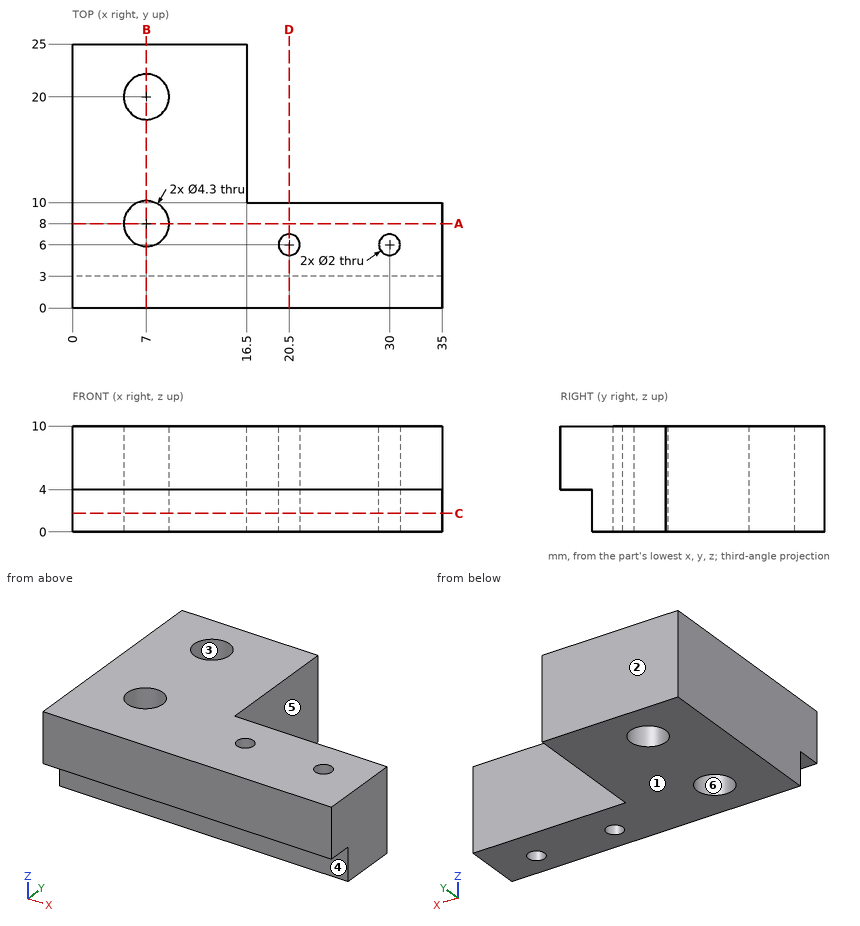
Geometry check sheet. Reference: drawing and pictorial views, mm from the part's lowest x, y, z. A direction names the side the tool comes from. Coordinates: 2 decimals unless noted, no trailing zeros. Order: outer loops, then holes, each group sorted by start corner. A loop starts at its lowest first (then second) coordinate and runs counter-clockwise, first axis right, second up.
Item 1: Section check A-A, the plane y = 8. Enter the section's corners in (x, z).
Filled in:
outline: (0, 0) - (4.85, 0) - (4.85, 10) - (0, 10) - close; (9.15, 0) - (35, 0) - (35, 10) - (9.15, 10) - close
Item 2: Material ranges on L1, parallel to Y at x = 7, z = 3; L2, parallel to Y at x = 30, z = 4.25; L3, parallel to Y at x = 8, z = 4.75, recorded low to high.
Filled in:
L1: y = 3 to 5.85, 10.15 to 17.85, 22.15 to 25
L2: y = 0 to 5, 7 to 10
L3: y = 0 to 6.1, 9.9 to 18.1, 21.9 to 25
Item 3: Section check B-B, the plane x = 7. Enter the section's corners in (y, z), then the cut area to 3 significant figures.
Filled in:
outline: (0, 4) - (3, 4) - (3, 0) - (5.85, 0) - (5.85, 10) - (0, 10) - close; (10.15, 0) - (17.85, 0) - (17.85, 10) - (10.15, 10) - close; (22.15, 0) - (25, 0) - (25, 10) - (22.15, 10) - close
area: 152 mm2
Item 4: Section check D-D, the plane x = 20.5. Enter the section's corners in (y, z).
Filled in:
outline: (0, 4) - (3, 4) - (3, 0) - (5, 0) - (5, 10) - (0, 10) - close; (7, 0) - (10, 0) - (10, 10) - (7, 10) - close
Item 5: Section check C-C, the plane z = 1.75. Enter the section's corners in (x, y), then the cut area to 3 significant figures.
Filled in:
outline: (0, 3) - (35, 3) - (35, 10) - (16.5, 10) - (16.5, 25) - (0, 25) - close; hole circle Ø4.3 at (7, 8); hole circle Ø4.3 at (7, 20); hole circle Ø2 at (20.5, 6); hole circle Ø2 at (30, 6)
area: 457 mm2
Item 6: Depth check by flat-ended pin: pin 1 (4.5 mm diameter, centred on x = 12, z = 1.5, fed in from -Y); pin 2 (4 mm diameter, centred on x = 7, y = 8, fed in from +Z); pin 3 (5 mm diameter, centred on y = 18.5, z = 8.5, fed in from +X); pin 4 (1.5 mm diameter, centred on x = 20, y = 2, fed in from -Z). Enter the tip coordinate at first touch or a pass-through.
Filled in:
pin 1: stops at y = 3
pin 2: passes through
pin 3: stops at x = 16.5
pin 4: stops at z = 4
Item 7: Access from +Z, -Z, +X, -X, +Y, -Y to the whole of each face (thin tool, end or side, straight path). Record for the marked faces 4, 5 and 6.
Filled in:
face 4: -Z, +X, -X, -Y
face 5: +Z, -Z, +X, +Y
face 6: +Z, -Z
Item 8: Release check for a two-part mould opening along Y. For the marked faces 1, 2 and 3 record: +Y half, -Y half, draft (parallel to the pull), parting line (faces both ways), or undercut.
Filled in:
face 1: draft
face 2: +Y half
face 3: undercut
